Read the model definition and answer for the solid it produces. Units are mm, in the model's axes. A direction names the side the tool comes from. Give positions to 0.01 mm unless a question says otherwise; leave off trailing zeros. Write each loop counter-clockwise with the first axis right and the second up, starting at its lowest first coordinate (ties: lowest second). Pieces come first, ordered by that corner, then holes. Notation, with made-up numbers: M 12,63.25 L 67,63.25 A12 cw 67,75.25 Z; hole C 50,6 d1. An arc over 180 degrees is marked long. Answer as CSV lines item,"result". Start each with the question number.
Autodesk Inventor part; units mm, degrees
ref_plane "Work Plane1" through (-127, 0, 0) normal (1, 0, 0) x (0, 1, 0)
ref_plane "XZ Plane" through (0, 0, 0) normal (0, 1, 0) x (-1, 0, 0)
ref_plane "XY Plane" through (0, 0, 0) normal (0, 0, 1) x (1, 0, 0)
sketch "Sketch1" plane through (0, 0, 0) normal (0, 0, 1) x (1, 0, 0)
  circle A0 centre (0, 0) radius 127
  dimension "d0" = 254
extrude "Extrusion1" add sketch "Sketch1" along normal blind 1828.8
ref_plane "Work Plane1" through (-127, 0, 0) normal (1, 0, 0) x (0, 1, 0)
sketch "Sketch2" plane through (0, 0, 0) normal (0, 0, -1) x (-1, 0, 0)
  circle A0 centre (0, 0) radius 101.6
  dimension "d3" = 203.2
extrude "Extrusion2" cut sketch "Sketch2" against normal blind 304.8
sketch "Sketch3" plane through (-127, 0, 0) normal (1, 0, 0) x (0, 1, 0)
  circle A0 centre (0, 152.4) radius 12.7
  point P0 (0, 0)
  dimension "d6" = 25.4
  dimension "d7" = 152.4
hole "Hole1" at (-127, 0, 152.4) direction (1, 0, 0) diameter 21.971 end through all
properties part number "OuterRadiusPoleAJB"
1. Find section B-B on y = -30.5. Determine the outline of the cut face in (x, z).
2. Find section A-A on x = 0. Determine the outline of the cut face in (y, z), then the cut area to 3 significant figures.
3. Given pin 1 (13 mm diameter, centred on y = 0, z = 152.4, fed in from -X); pin 2 (1 mm diameter, centred on y = -77, z = 765, fed in from -X); pin 3 (6 mm diameter, centred on y = 7, z = 624.5, fed in from +X); pin 4 (10 mm diameter, centred on x = 76.5, z = 348.5, fed in from +Y), each flat-ended and moving along its own axis, determine where each tip first touches the part or whether it passes through.
4. Find section C-C on z = 1601.5. Determine the outline of the cut face in (x, y), then the cut area to 3 significant figures.
5. Find the intervals of material crossed by line 1 (Z direction, x = 116, y = 0); line 2 (X direction, y = 0, z = 118); line 3 (Y direction, x = -9, z = 1337), in increasing order. Write a range as [from, to].
6. Determine the mould class of faces 1 (the face through (1, 1, 304.8)), 2 (the face through (-57, 85, 0)), 3 (the face through (-27.53, 123.98, 901.6)) for opening direction Y: +Y half, -Y half, draft (parallel to the pull), parting line (faces both ways), or undercut.
7. For faces 4 (the face through (-2, 2, 1828.8)), 5 (the face through (-96.908, 30.518, 150.266)), determine the directions among +Z, -Z, +X, -X, +Y, -Y from which every point of the face is accessible in a straight line to the end or side of a thin tool.
Computed:
1,outline,"M -123.28,0 L -96.91,0 L -96.91,304.8 L 96.91,304.8 L 96.91,0 L 123.28,0 L 123.28,1828.8 L -123.28,1828.8 Z"
2,outline,"M -127,0 L -101.6,0 L -101.6,304.8 L 101.6,304.8 L 101.6,0 L 127,0 L 127,1828.8 L -127,1828.8 Z"
2,area,"403,000 mm^2"
3,pin 1,"passes through"
3,pin 2,"stops at x = -101.37"
3,pin 3,"stops at x = 126.94"
3,pin 4,"stops at y = 104.96"
4,outline,"C 0,0 d254"
4,area,"50,700 mm^2"
5,line 1,"z = [0, 141.41], [163.39, 1828.8]"
5,line 2,"x = [-127, -101.6], [101.6, 127]"
5,line 3,"y = [-126.68, 126.68]"
6,face 1,"undercut"
6,face 2,"draft"
6,face 3,"parting line"
7,face 4,"+Z, +X, -X, +Y, -Y"
7,face 5,"-Z"
